Part print with two shaded views. Sizes in mm from the minimum x, y, z corner. A direction names the side the tool comes from. Round coordinates to 2 decimals unless told otherwise and drop trailing zeros. Write each loop counter-clockwise with the first axis right and the second up, starting at its lowest first coordinate (ties: lowest second). Pieces come first, ordered by that corner, then holes. Notation, with made-up numbers: (87.5, 68.5) -> (142.5, 68.5) arc R25 cw to (142.5, 107.5) -> close; hole circle Ø9 at (-17.75, 74). An arc over 180 degrees is marked (long way). Answer as CSV lines item,"result".
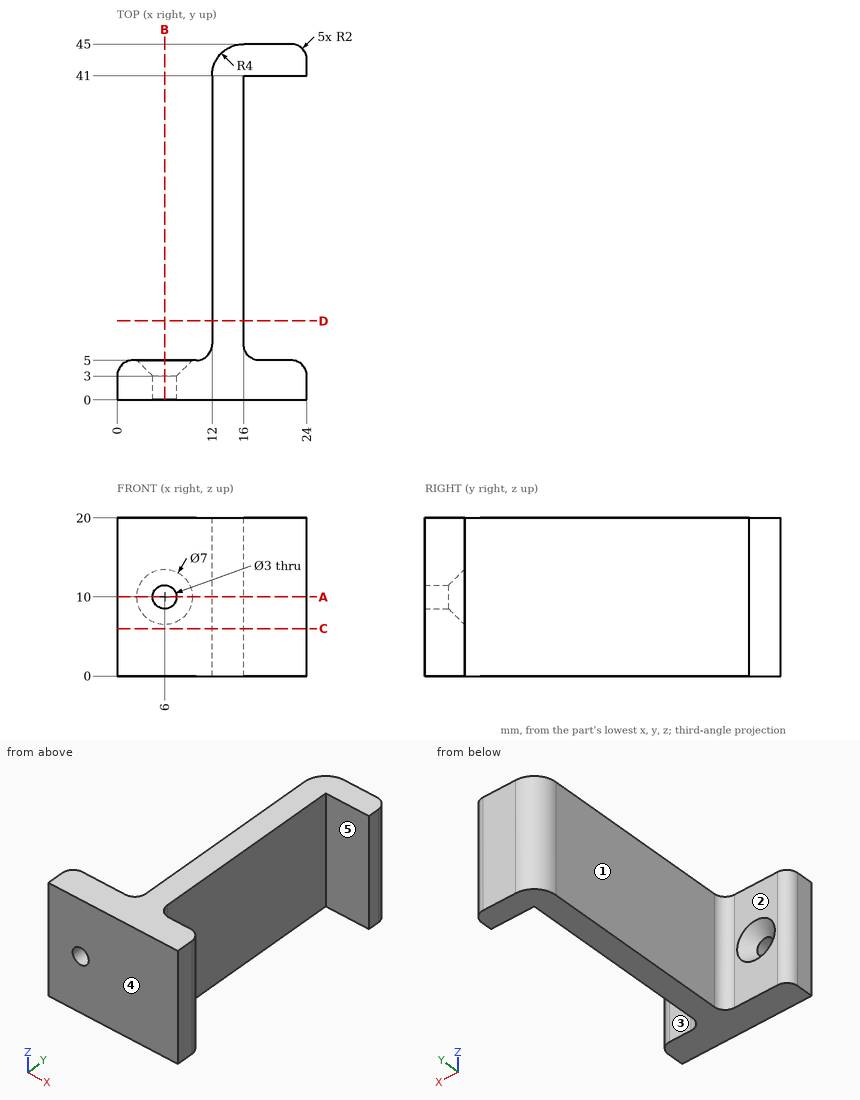
1. Cut at C-C, the plane z = 6. Write the cut outline in (x, y).
Results found:
outline,"(0, 0) -> (24, 0) -> (24, 3) arc R2 ccw to (22, 5) -> (18, 5) arc R2 cw to (16, 7) -> (16, 41) -> (24, 41) -> (24, 43) arc R2 ccw to (22, 45) -> (16, 45) arc R4 ccw to (12, 41) -> (12, 7) arc R2 cw to (10, 5) -> (2, 5) arc R2 ccw to (0, 3) -> close"
2. Probe line 1 along X through (y, z) = (1.05, 10); line 2 along Z through (x, y) = (6, 2.15); line 3 along Y through (x, z) = (19.5, 5.25). List the from-to ranges inside material, lowest first.
Results found:
line 1,"x = 0 to 4.5, 7.5 to 24"
line 2,"z = 0 to 8.5, 11.5 to 20"
line 3,"y = 0 to 5, 41 to 45"
3. Cut at B-B, the plane x = 6. Write the cut outline in (y, z).
Results found:
outline,"(0, 0) -> (5, 0) -> (5, 6.5) -> (3, 8.5) -> (0, 8.5) -> close; (0, 11.5) -> (3, 11.5) -> (5, 13.5) -> (5, 20) -> (0, 20) -> close"
4. Drop flat-ended pins along their axis: pin 1 Ø6.5 at (x, z) = (8, 10.5) entering from +Y; pin 2 Ø6 at (x, z) = (4, 3) entering from +Y; pin 3 Ø1 at (y, z) = (32.5, 14) entering from +X; pin 4 Ø2.5 at (x, z) = (6, 10) entering from +Y. Give the stop position or say it passes through.
Results found:
pin 1,"stops at y = 5.44"
pin 2,"stops at y = 5"
pin 3,"stops at x = 16"
pin 4,"passes through"
5. Cut at A-A, the plane z = 10. Write the cut outline in (x, y), then the cut area to 3 significant figures.
Results found:
outline,"(0, 0) -> (4.5, 0) -> (4.5, 3) -> (2.5, 5) -> (2, 5) arc R2 ccw to (0, 3) -> close; (7.5, 0) -> (24, 0) -> (24, 3) arc R2 ccw to (22, 5) -> (18, 5) arc R2 cw to (16, 7) -> (16, 41) -> (24, 41) -> (24, 43) arc R2 ccw to (22, 45) -> (16, 45) arc R4 ccw to (12, 41) -> (12, 7) arc R2 cw to (10, 5) -> (9.5, 5) -> (7.5, 3) -> close"
area,"289 mm2"
6. Which spindle directions (+Z, -Z, +X, -X, +Y, -Y) get a long thin tool onto all of the face, cutting with end or side? Do the marked faces 4 and 5. Say none if no direction does.
Results found:
face 4,"+Z, -Z, +X, -X, -Y"
face 5,"+Z, -Z, +X"
7. Cut at D-D, the plane y = 10. Write the cut outline in (x, z).
Results found:
outline,"(12, 0) -> (16, 0) -> (16, 20) -> (12, 20) -> close"
8. Mould opens along Y. For the marked faces 1, 2 and 3 say: +Y half, -Y half, draft (parallel to the pull), parting line (faces both ways), or undercut.
Results found:
face 1,"draft"
face 2,"+Y half"
face 3,"undercut"
